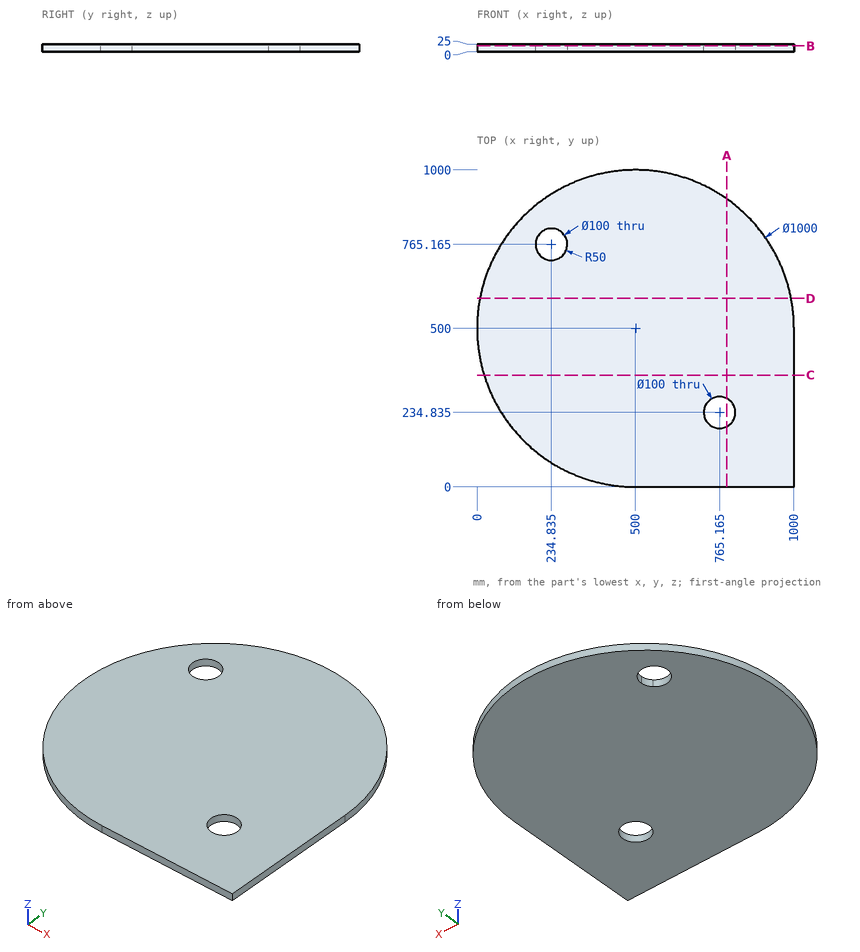
Can you work these out from the drawing? Everything is in mm from the part's minimum corner. Round coordinates to 2 decimals unless told otherwise and drop trailing zeros. Order: outer loops, then holes, each group sorted by start corner. A loop starts at its lowest first (then second) coordinate and runs counter-clockwise, first axis right, second up. Notation, with made-up numbers: (4, 16.5) - (12, 16.5) arc R7 ccw to (12, 29.5) - close; hole circle Ø8 at (22, 61.25). An arc over 180 degrees is marked (long way). Answer in a Markdown table with one row per item.
(1) Please list where these lines run through material, in increasing order: L1, parallel to X at y = 783, z = 3.5; L2, parallel to Y at x = 243.5, z = 11.75; L3, parallel to X at y = 496.5, z = 12.25. Write a range as from..to.
From the geometry:
| item | result |
|---|---|
| L1 | x = 87.8..188.12, 281.55..912.2 |
| L2 | y = 70.81..715.92, 814.41..929.19 |
| L3 | x = 0.01..1000 |
(2) For P1, Ø10, axis at y = 237.5, z = 15.5, coming from the -X side (3 decimals); P2, Ø10, axis at y = 824.5, z = 13, coming from the -X side; P3, Ø1, axis at y = 105, z = 17.5, coming from the -X side; P4, Ø4, axis at x = 771, y = 757, coming from the -Z side, each with a flat end and sliding along its axis, tell me the tip position at first contact or that it passes through.
From the geometry:
| item | result |
|---|---|
| P1 | stops at x = 71.405 |
| P2 | stops at x = 115.4 |
| P3 | stops at x = 192.8 |
| P4 | stops at z = 0 |
(3) Suppose I cut it at C-C, the plane y = 352.5. Please give me the cut outline in (x, z), plus the area to 3 significant figures.
From the geometry:
| item | result |
|---|---|
| outline | (22.25, 0) - (1000, 0) - (1000, 25) - (22.25, 25) - close |
| area | 24,400 mm2 |
(4) Suppose I cut it at A-A, the plane x = 788. Please give me the cut outline in (y, z).
From the geometry:
| item | result |
|---|---|
| outline | (0, 0) - (190.35, 0) - (190.35, 25) - (0, 25) - close; (279.32, 0) - (908.72, 0) - (908.72, 25) - (279.32, 25) - close |
(5) Suppose I cut it at D-D, the plane y = 594.5. Please give me the cut outline in (x, z), plus the area to 3 significant figures.
From the geometry:
| item | result |
|---|---|
| outline | (9.01, 0) - (990.99, 0) - (990.99, 25) - (9.01, 25) - close |
| area | 24,500 mm2 |
(6) Suppose I cut it at B-B, the plane z = 19.25. Please give me the cut outline in (x, y) (3 decimals), plus the area to 3 significant figures.
From the geometry:
| item | result |
|---|---|
| outline | (500, 0) - (1000, 0) - (1000, 500) arc R500 ccw (long way) to start; hole (270.19, 729.81) arc R50 ccw to (284.835, 765.165) arc R50 ccw (long way) to start; hole circle Ø100 at (765.165, 234.835) |
| area | 823,000 mm2 |
